Can you work these out from the model? Positions are in its coordinate system, mm. Face numbers are marked on the shaded views. A direction names the side the tool comes from. Give positions to 0.01 mm unless a question says otherwise; leave off trailing zeros. Loops run counter-clockwise (first coordinate to the right, second up) from the corner with the lowest first, then second, coordinate; pieces in that order, holes last. Notation, with made-up numbers: (-35, -26) - (15, -26) arc R37 ccw to (15, 10) - close; hole circle Ø4 at (1, -34). An arc over 180 degrees is marked (long way). Answer in a Markdown table with one row per item.
from build123d import *

# Parameters (mm, degrees)
BOSS_EXTRU_1_DEPTH      = 3
BOSS_EXTRU_2_DEPTH      = 6
ENL_V_MAT_EXTRU_1_DEPTH = 6


with BuildPart() as part:
    # Esquisse1 → Boss.-Extru.1 (new body, symmetric)
    with BuildSketch(Plane(origin=(0, 0, 0), x_dir=(0, -1, 0), z_dir=(1, 0, 0))):
        Polygon((0, 0), (42, 42), (47, 42), (47, -5), (0, -5), align=None)
    extrude(amount=BOSS_EXTRU_1_DEPTH, both=True)

    # Esquisse2 → Boss.-Extru.2 (add)
    with BuildSketch(Plane(origin=(3, 0, 0), x_dir=(0, -1, 0), z_dir=(1, 0, 0))):
        with BuildLine():
            Line((14.5, -10), (14.5, -5))
            Line((14.5, -5), (6.5, -5))
            Line((6.5, -5), (6.5, -10))
            ThreePointArc((6.5, -10), (6.792893219, -10.707106781), (7.5, -11))
            Line((7.5, -11), (13.5, -11))
            ThreePointArc((13.5, -11), (14.207106781, -10.707106781), (14.5, -10))
        make_face()
        with BuildLine():
            Line((37.5, -10), (37.5, -5))
            Line((37.5, -5), (29.5, -5))
            Line((29.5, -5), (29.5, -10))
            ThreePointArc((29.5, -10), (29.792893219, -10.707106781), (30.5, -11))
            Line((30.5, -11), (36.5, -11))
            ThreePointArc((36.5, -11), (37.207106781, -10.707106781), (37.5, -10))
        make_face()
        with BuildLine():
            Line((52, 12.5), (47, 12.5))
            Line((47, 12.5), (47, 4.5))
            Line((47, 4.5), (52, 4.5))
            ThreePointArc((52, 4.5), (52.707106781, 4.792893219), (53, 5.5))
            Line((53, 5.5), (53, 11.5))
            ThreePointArc((53, 11.5), (52.707106781, 12.207106781), (52, 12.5))
        make_face()
        with BuildLine():
            Line((52, 35.5), (47, 35.5))
            Line((47, 35.5), (47, 27.5))
            Line((47, 27.5), (52, 27.5))
            ThreePointArc((52, 27.5), (52.707106781, 27.792893219), (53, 28.5))
            Line((53, 28.5), (53, 34.5))
            ThreePointArc((53, 34.5), (52.707106781, 35.207106781), (52, 35.5))
        make_face()
    extrude(amount=-BOSS_EXTRU_2_DEPTH)

    # Esquisse2_3 → Enl_v. mat.-Extru.1 (cut)
    with BuildSketch(Plane(origin=(3, 0, 0), x_dir=(0, -1, 0), z_dir=(1, 0, 0))):
        Polygon((19.5, -5), (24.5, -5), (24.5, 0), (26.3, 0), (26.3, 5.5), (24.5, 5.5), (24.5, 9.5), (19.5, 9.5), (19.5, 5.5), (17.7, 5.5), (17.7, 0), (19.5, 0), align=None)
        Polygon((47, 17.5), (47, 22.5), (42, 22.5), (42, 24.3), (36.5, 24.3), (36.5, 22.5), (32.5, 22.5), (32.5, 17.5), (36.5, 17.5), (36.5, 15.7), (42, 15.7), (42, 17.5), align=None)
    extrude(amount=-ENL_V_MAT_EXTRU_1_DEPTH, mode=Mode.SUBTRACT)


solid = part.part
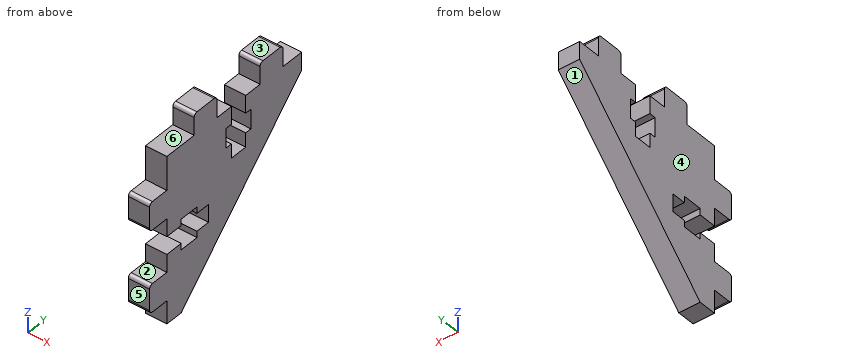
Q1. On a 3-axis mill with a long thin cutter (end or side, diameter ignored), from which of +Z, -Z, +X, -X, +Y, -Y can I reach the whole of each face in a straight line? I mean the marked faces 5 and 6. Say none if no direction works.
Checked values:
| item | result |
|---|---|
| face 5 | +Z, -Z, +X, -X, -Y |
| face 6 | +Z, +X, -X, -Y |
Q2. Imagine slicing it at D-D, the plane y = -22.5. Write out the boundary of the cut face in (x, z), and give its area (3 significant figures).
Checked values:
| item | result |
|---|---|
| outline | (-3, -22.5) - (3, -22.5) - (3, -9.5) - (-3, -9.5) - close |
| area | 78.0 mm² |
Q3. If I drill on line 1 (Y direction, x = -1.2, z = -6.5); line 2 (Z direction, x = 0.95, y = -49); line 3 (Y direction, x = -2.2, z = 8), over which ranges is the centre line in solid material (lowest first)? Write a range as [from, to].
Checked values:
| item | result |
|---|---|
| line 1 | y = [-53, -24.5], [-19.5, -6.5] |
| line 2 | z = [-35.5, -27.5], [-12.5, -4.5] |
| line 3 | y = [-37.5, -29.5], [-14.5, -6.5] |
Q4. Imagine slicing it at C-C, the plane z = -20.5. Write out the boundary of the cut face in (x, y).
Checked values:
| item | result |
|---|---|
| outline | (-3, -32.5) - (3, -32.5) - (3, -20.5) - (-3, -20.5) - close |
Q5. Imagine slicing it at A-A, the plane y = -34. Write out the boundary of the cut face in (x, z).
Checked values:
| item | result |
|---|---|
| outline | (-3, -34) - (3, -34) - (3, -22.5) - (-3, -22.5) - close; (-3, -17.5) - (3, -17.5) - (3, 11) - (-3, 11) - close |
Q6. If we mould it in two halves opening along Z, with no side actions, what happens to the marked faces 1, 2, 3 and 4? For each: released by +Z, released by -Z, zero draft, split by the parting line, or undercut.
Checked values:
| item | result |
|---|---|
| face 1 | released by -Z |
| face 2 | undercut |
| face 3 | released by +Z |
| face 4 | zero draft |
Q7. For pin 1 (2.5 mm diameter, centred on x = 0, z = 1.5, fed in from -Y); pin 2 (2.5 mm diameter, centred on x = 1, z = 8.5, fed in from +Y); pin 3 (2.5 mm diameter, centred on x = -0.5, z = 7.5, fed in from -Y), each with a flat end and sliding along its axis, tell me the tip position at first contact or that it passes through.
Checked values:
| item | result |
|---|---|
| pin 1 | stops at y = -47 |
| pin 2 | stops at y = -6.5 |
| pin 3 | stops at y = -37.5 |
Q8. Imagine slicing it at B-B, the plane z = -3. Write out the boundary of the cut face in (x, y).
Checked values:
| item | result |
|---|---|
| outline | (-3, -47) - (3, -47) - (3, -26.3) - (-3, -26.3) - close; (-3, -17.7) - (3, -17.7) - (3, -3) - (-3, -3) - close |
